The drawing under review shows one solid part. Ordinate dimensions are in mm from its lowest x, y, z. A direction names the side the tool comes from. Give positions to 0.01 mm unless a question says otherwise; leave off trailing zeros. Loops run counter-clockwise (first coordinate to the right, second up) from the corner with the lowest first, then second, coordinate; pieces in that order, holes last. Notation, with made-up numbers: M 53.5,14.5 L 72.5,14.5 A10 ccw 72.5,25.5 Z; hole C 13,85.5 d11. An arc over 180 degrees is marked long. One line per item, written item: value. Start each with the question number.
Q1. We need section C-C on y = 2. Write out the cut boundary in (x, z).
Q2. To check wall thickness, follow line 1 along X through (y, z) = (20, 3.5); line 2 along Y through (x, z) = (50, 3); line 3 along Y through (x, z) = (49, 17). State the ranges of each line that lie inside material, in increasing order. Write a range as from..to.
Q3. For the marked faces 1 and 2, list the 3-axis set-ups (+Z, -Z, +X, -X, +Y, -Y) from which the entire face can be reached by the end or side of a thin tool; tool diameter is ignored.
Q4. We need section D-D on x = 8. Write out the cut boundary in (y, z), plus the area to 3 significant figures.
Q5. For pin 1 (17.5 mm diameter, centred on x = 33.5, y = 20.5, fed in from +Z); pin 2 (2 mm diameter, centred on x = 22, z = 16, fed in from +Y), all flat-tipped, find the tip position at first contact; note any pin that passes through.
Q6. We need section B-B on z = 23. Write out the cut boundary in (x, y), plus the area to 4 significant figures.
Q7. Mouldability with a two-part tool opening along Z and no side actions: class the marked faces 3, 4 and 5 as released by +Z, released by -Z, zero draft, split by the parting line, or undercut.
Q8. We need section A-A on x = 50. Write out the cut boundary in (y, z).
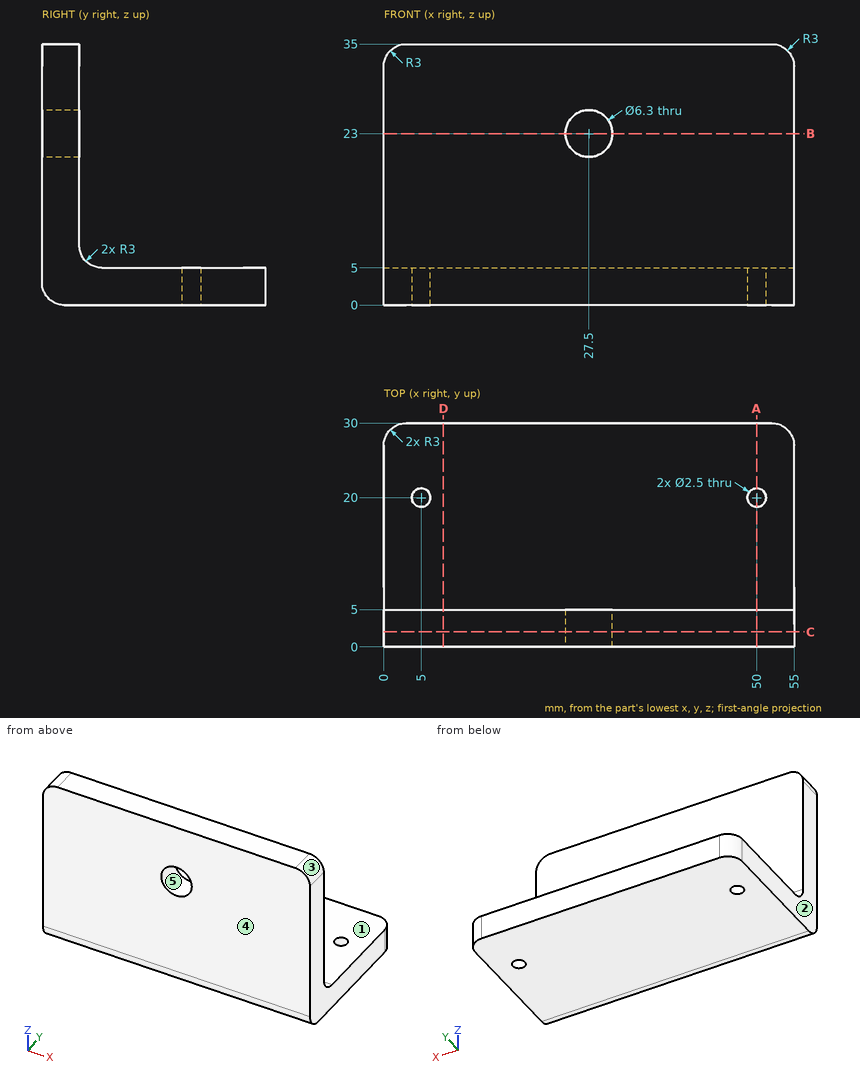
Solved:
1. outline: M 0,0.17 L 55,0.17 L 55,32 A3 ccw 52,35 L 3,35 A3 ccw 0,32 Z; hole C 27.5,23 d6.3
2. line 1: 0..3.75, 6.25..48.75, 51.25..55
2. line 2: 0..18.75, 21.25..30
2. line 3: 0..5
3. face 1: +Z, +X, -X, +Y
3. face 2: +Z, -Z, -X, +Y, -Y
4. outline: M 0,3 A3 ccw 3,0 L 30,0 L 30,5 L 8,5 A3 cw 5,8 L 5,35 L 0,35 Z
4. area: 300 mm2
5. pin 1: z = 5
5. pin 2: y = 5
6. outline: M 0,0 L 24.35,0 L 24.35,5 L 0,5 Z; M 30.65,0 L 55,0 L 55,5 L 30.65,5 Z
6. area: 243.5 mm2
7. face 3: released by +Z
7. face 4: zero draft
7. face 5: undercut
8. outline: M 0,3 A3 ccw 3,0 L 18.75,0 L 18.75,5 L 8,5 A3 cw 5,8 L 5,35 L 0,35 Z; M 21.25,0 L 30,0 L 30,5 L 21.25,5 Z
